Part model, mm, in its own coordinate system. Face numbers are marked on the shaded views. A direction names the side the tool comes from. Round coordinates to 2 decimals unless told otherwise and drop trailing zeros. Loops run counter-clockwise (first coordinate to the right, second up) from the corner with the lowest first, then second, coordinate; pieces in that order, holes last. Notation, with made-up numbers: M 19,-30 L 68,-30 A8 ccw 68,-20 Z; hole C 32,20.5 d11. An arc over 180 degrees is marked long. Put each result on its own line as item: value. Start each with the question number.
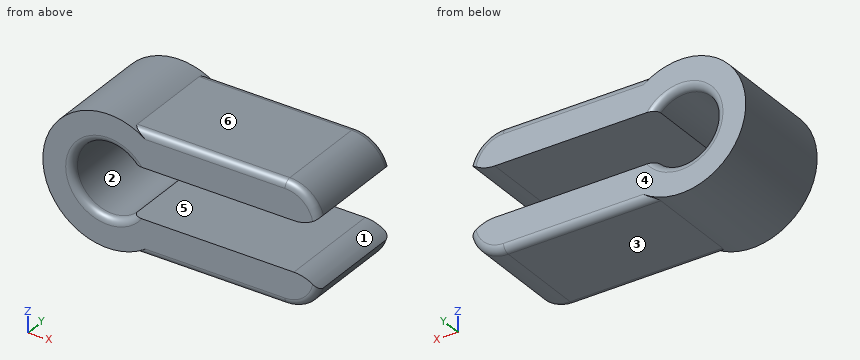
```python
from build123d import *

# Parameters (mm, degrees)
F1_DEPTH    = 15
F2_T1_DEPTH = 56.5812984693
F3_R        = 1


# Not quite as in the source:
# - a fillet or chamfer that OpenCascade refuses, or shapes differently, is made with other operations: its cross-section is extruded or revolved along the edge and cut away or added


with BuildPart() as f1:
    # F0 (on Front) → F1 (new body)
    with BuildSketch(Plane.XZ):
        with BuildLine():
            Line((30.5210083783, 8.55), (0.5210083783, 8.55))
            ThreePointArc((0.5210083783, 8.55), (-12.2466210045, 0), (0.5210083783, -8.55))
            Line((0.5210083783, -8.55), (30.5210083783, -8.55))
            Line((30.5210083783, -8.55), (26.9854744724, -5.0144660941))
            ThreePointArc((26.9854744724, -5.0144660941), (25.3633577283, -3.9306023374), (23.4499405664, -3.55))
            Line((23.4499405664, -3.55), (0.5210083783, -3.55))
            ThreePointArc((0.5210083783, -3.55), (-8, 0), (0.5210083783, 3.55))
            Line((0.5210083783, 3.55), (23.4499405664, 3.55))
            ThreePointArc((23.4499405664, 3.55), (25.3633577283, 3.9306023374), (26.9854744724, 5.0144660941))
            Line((26.9854744724, 5.0144660941), (30.5210083783, 8.55))
        make_face()
    extrude(amount=F1_DEPTH)

    # F2: fillet of radius 5 on 2 edges, made by hand

    # F2_s2 → F2_t1 (cut)
    with BuildSketch(Plane.XZ.offset(-20.7906492346)):
        with BuildLine():
            ThreePointArc((22.2047486844, -8.55), (25.1777664719, -7.5700951774), (26.9854744724, -5.0144660941))
            Line((26.9854744724, -5.0144660941), (30.5210083783, -8.55))
            Line((30.5210083783, -8.55), (22.2047486844, -8.55))
        make_face()
        with BuildLine():
            ThreePointArc((26.9854744724, 5.0144660941), (25.1777664719, 7.5700951774), (22.2047486844, 8.55))
            Line((22.2047486844, 8.55), (30.5210083783, 8.55))
            Line((30.5210083783, 8.55), (26.9854744724, 5.0144660941))
        make_face()
    extrude(amount=F2_T1_DEPTH, mode=Mode.SUBTRACT)

    # F3
    f3_edges = [f1.edges().sort_by_distance(p)[0] for p in [
        (11.362879, 0, -8.55),
        (11.362879, -15, -8.55),
        (11.362879, -15, 8.55),
        (11.362879, 0, 8.55),
        (-8, -15, 0),
        (-8, 0, 0),
        (25.177766, 0, 7.570095),
        (25.177766, -15, 7.570095),
        (25.177766, 0, -7.570095),
        (25.177766, -15, -7.570095),
    ]]
    fillet(f3_edges, radius=F3_R)


solid = f1.part
```
1. Cut at C-C, the plane z = 0. Give the cut face in (x, y).
2. Mould opens along X. For the marked faces 1, 2 and 3 say: released by +X, released by -X, zero draft, split by the parting line, or undercut.
3. Which spindle directions (+Z, -Z, +X, -X, +Y, -Y) get a long thin tool onto all of the face, cutting with end or side? Do the marked faces 4, 5 and 6. Say none if no direction does.
4. Cut at A-A, the plane x = 10. Give the cut face in (y, z).
5. Cut at B-B, the plane y = -12.75. Give the cut face in (x, z), and give its area (3 significant figures).
6. Wall check: L1, parallel to Z at x = -3, y = -7.25; L2, parallel to Z at x = 4, y = -9.5; L3, parallel to X at y = -3.75, z = 0. Give the ranges that are in metal, low to high.
7. Drop flat-ended pins along their axis: pin 1 (3 mm diameter, centred on x = 5.5, y = -5, fed in from +Z); pin 2 (9 mm diameter, centred on x = -3, z = 0, fed in from -Y); pin 3 (6 mm diameter, centred on y = -9, z = 1.5, fed in from +X); pin 4 (8 mm diameter, centred on x = 7, y = -13, fed in from -Z). Give the stop position or say it passes through.
Results list:
1. outline: M -12.25,-15 L -9,-15 A1 ccw -8,-14 L -8,-1 A1 ccw -9,0 L -12.25,0 Z
2. face 1: released by +X
2. face 2: undercut
2. face 3: zero draft
3. face 4: +Z, -Z, +X, -X, +Y
3. face 5: +X, +Y, -Y
3. face 6: +Z, +X, +Y, -Y
4. outline: M -15,-7.55 A1 ccw -14,-8.55 L -1,-8.55 A1 ccw 0,-7.55 L 0,-3.55 L -15,-3.55 Z; M -15,3.55 L 0,3.55 L 0,7.55 A1 ccw -1,8.55 L -14,8.55 A1 ccw -15,7.55 Z
5. outline: M 0.52,-8.55 L 22.2,-8.55 A5 ccw 26.99,-5.01 A5 ccw 23.45,-3.55 L 0.52,-3.55 A5 cw long 0.52,3.55 L 23.45,3.55 A5 ccw 26.99,5.01 A5 ccw 22.2,8.55 L 0.52,8.55 A9.25 ccw long Z
5. area: 379 mm^2
6. L1: z = -9.25 to -5, 5 to 9.25
6. L2: z = -8.55 to -3.55, 3.55 to 8.55
6. L3: x = -12.25 to -8
7. pin 1: stops at z = 8.55
7. pin 2: passes through
7. pin 3: stops at x = 26.38
7. pin 4: stops at z = -8.55
